Geometry: final body of the model. Coordinates: model frame, mm. Give positions to 0.01 mm unless a question says otherwise; leave off trailing zeros. Loops run counter-clockwise (first coordinate to the right, second up) from the corner with the lowest first, then second, coordinate; pieces in that order, holes last.
1. Section A-A, the plane z = 25. Output: boundary loops of the cut face in (x, y).
2. Draft query along X for faces 1 (the face through (-5, -12, 0)), 2 (the face through (16.486, 19.297, 24.65)), 3 (the face through (11.923, 3.755, 24.65)). Return one class per face: +X half, -X half, draft (parallel to the pull), parting line (faces both ways), or undercut.
3. Section D-D, the plane x = 18.5. Output: boundary loops of the cut face in (y, z).
4. First-contact query: P1, Ø10, axis at x = 3, y = 5.5, coming from the +Z side; P2, Ø1, axis at y = 10, z = 8, coming from the -X side; P3, Ø5, axis at x = 11, z = 36.5, coming from the +Y side; P4, Ø1.5, axis at x = 4, z = 9, coming from the -Y side. Flat tips, straight axial feed; report the tip coordinate or a pass-through.
5. Section B-B, the plane x = 0. Output: boundary loops of the cut face in (y, z), then the cut area to 3 significant figures.
6. Material intervals for line 1 along Y through (x, z) = (0, 25); line 2 along Y through (x, z) = (1.5, 36); line 3 along Y through (x, z) = (-14.5, 13.5), sorted ascending.
7. Section C-C, the plane y = -30. Output: boundary loops of the cut face in (x, z), then the cut area to 4 significant figures.
from build123d import *

# Parameters (mm, degrees)
SKETCH1_R           = 12.5
BOSS_EXTRUDE1_DEPTH = 50
SKETCH2_R           = 12.5
BOSS_EXTRUDE2_DEPTH = 22.5


with BuildPart() as part:
    # Sketch1 → Boss-Extrude1 (new body)
    with BuildSketch(Plane.XY):
        with BuildLine():
            Line((-2.5, 25), (2.5, 25))
            ThreePointArc((2.5, 25), (16.642135624, 19.142135624), (22.5, 5))
            Line((22.5, 5), (22.5, -15))
            Line((22.5, -15), (-22.5, -15))
            Line((-22.5, -15), (-22.5, 5))
            ThreePointArc((-22.5, 5), (-16.642135624, 19.142135624), (-2.5, 25))
        make_face()
        Circle(SKETCH1_R, mode=Mode.SUBTRACT)
    extrude(amount=BOSS_EXTRUDE1_DEPTH)

    # Sketch2 → Boss-Extrude2 (add, symmetric)
    with BuildSketch(Plane(origin=(0, 0, 0), x_dir=(0, 0, -1), z_dir=(1, 0, 0))):
        with BuildLine():
            Line((-50, -15), (-50, -35))
            ThreePointArc((-50, -35), (-44.142135624, -49.142135624), (-30, -55))
            Line((-30, -55), (-20, -55))
            ThreePointArc((-20, -55), (-5.857864376, -49.142135624), (0, -35))
            Line((0, -35), (0, -15))
            Line((0, -15), (-50, -15))
        make_face()
        with Locations((-25, -30)):
            Circle(SKETCH2_R, mode=Mode.SUBTRACT)
    extrude(amount=BOSS_EXTRUDE2_DEPTH, both=True)


solid = part.part
Answers below:
1. outline: (-22.5, -55) - (22.5, -55) - (22.5, -42.5) - (-22.5, -42.5) - close; (-22.5, -17.5) - (22.5, -17.5) - (22.5, 5) arc R20 ccw to (2.5, 25) - (-2.5, 25) arc R20 ccw to (-22.5, 5) - close; hole circle Ø25 at (0, 0)
2. face 1: draft
2. face 2: +X half
2. face 3: undercut
3. outline: (-55, 20) arc R20 ccw to (-35, 0) - (17, 0) - (17, 50) - (-35, 50) arc R20 ccw to (-55, 30) - close; hole circle Ø25 at (-30, 25)
4. P1: passes through
4. P2: stops at x = -21.99
4. P3: stops at y = 24.08
4. P4: stops at y = -52.17
5. outline: (-55, 20) arc R20 ccw to (-35, 0) - (-12.5, 0) - (-12.5, 50) - (-35, 50) arc R20 ccw to (-55, 30) - close; (12.5, 0) - (25, 0) - (25, 50) - (12.5, 50) - close; hole circle Ø25 at (-30, 25)
5. area: 2,090 mm2
6. line 1: y = -55 to -42.5, -17.5 to -12.5, 12.5 to 25
6. line 2: y = -54.08 to -35.94, -24.06 to -12.41, 12.41 to 25
6. line 3: y = -53.91 to -34.9, -25.1 to 21
7. outline: (-22.5, 0) - (22.5, 0) - (22.5, 12.5) - (-22.5, 12.5) - close; (-22.5, 37.5) - (22.5, 37.5) - (22.5, 50) - (-22.5, 50) - close
7. area: 1,125 mm2
